from build123d import *

# Parameters (mm, degrees)
SZKIC1_R                    = 2.1
DODANIE_WYCI_GNI_CIE1_DEPTH = 24
WYTNIJ_WYCI_GNI_CIE1_REACH  = 31.306
SZKIC3_R                    = 3.45
WYTNIJ_WYCI_GNI_CIE2_DEPTH  = 4


with BuildPart() as part:
    # Szkic1 → Dodanie-wyciągnięcie1 (new body)
    with BuildSketch(Plane(origin=(0, 0, 0), x_dir=(1, 0, 0), z_dir=(0, 1, 0))):
        Polygon((12.5, 3.9), (-12.5, 3.9), (-14.9, 1.5), (-14.9, -1.5), (-12.5, -3.9), (12.5, -3.9), (14.9, -1.5), (14.9, 1.5), align=None)
        with Locations(Location((-11, 0, 0), (0, 0, 270))):
            Circle(SZKIC1_R, mode=Mode.SUBTRACT)
        with Locations(Location((11, 0, 0), (0, 0, 90))):
            Circle(SZKIC1_R, mode=Mode.SUBTRACT)
    extrude(amount=-DODANIE_WYCI_GNI_CIE1_DEPTH)

    # Szkic2 → Wytnij-wyciągnięcie1 (cut, up to next)
    with BuildSketch(Plane(origin=(0, 0, -3.9), x_dir=(-1, 0, 0), z_dir=(0, 0, -1)), mode=Mode.PRIVATE) as wytnij_wyci_gni_cie1_sk1:
        with BuildLine():
            Line((-7.1, -24), (7.1, -24))
            ThreePointArc((7.1, -24), (0, -16.9), (-7.1, -24))
        make_face()
    wytnij_wyci_gni_cie1_tool1 = extrude(wytnij_wyci_gni_cie1_sk1.sketch, amount=-WYTNIJ_WYCI_GNI_CIE1_REACH, mode=Mode.PRIVATE) & part.part
    add(wytnij_wyci_gni_cie1_tool1.solids().sort_by_distance((0, -20.986666, -3.9))[0], mode=Mode.SUBTRACT)

    # Szkic3 → Wytnij-wyciągnięcie2 (cut)
    with BuildSketch(Plane(origin=(0, 0, 0), x_dir=(1, 0, 0), z_dir=(0, 1, 0))):
        with Locations(Location((-11, 0, 0), (0, 0, 270))):
            Circle(SZKIC3_R)
        with Locations(Location((11, 0, 0), (0, 0, 90))):
            Circle(SZKIC3_R)
    extrude(amount=-WYTNIJ_WYCI_GNI_CIE2_DEPTH, mode=Mode.SUBTRACT)


solid = part.part
CAD build for the part. Positions are in the model's coordinates, mm. A direction names the side the tool comes from. Give positions to 0.01 mm unless a question says otherwise; leave off trailing zeros. Loops run counter-clockwise (first coordinate to the right, second up) from the corner with the lowest first, then second, coordinate; pieces in that order, holes last. Notation, with made-up numbers: M -8,35.5 L 25,35.5 A31 ccw 25,66.5 Z; hole C 69,40.5 d4. An arc over 180 degrees is marked long. One line per question, with ' | ' between items. Start each with the question number.
1. Probe L1, parallel to X at y = -2.85, z = 0; L2, parallel to X at y = -11.5, z = 0; L3, parallel to X at y = -19, z = 0. List the from-to ranges inside material, lowest first. Write a range as from..to.
2. Saw through at A-A on z = 0. Give the cut face in (x, y).
3. Saw through at B-B on x = 11. Give the cut face in (y, z), plus the area to 3 significant figures.
4. Saw through at D-D on x = -5. Give the cut face in (y, z), plus the area to 3 significant figures.
5. Two-plate mould, pull along Z, no slides. Class faces 1 (the face through (8.918, -13.86, 0.273)), 2 (the face through (13.7, -11.8, 2.7)), 3 (the face through (13.7, -11.8, -2.7)): pulls with the +Z half, pulls with the -Z half, needs draft (parallel to the pull), parting line crosses it, or undercut.
6. Flat gauge pins, fed straight in: pin 1 (1 mm diameter, centred on y = -17, z = -3, fed in from +X); pin 2 (2 mm diameter, centred on x = -11, z = 1.5, fed in from +Y); pin 3 (2.5 mm diameter, centred on x = 11, z = 0, fed in from +Y). Where does each tip first touch, or does it go through?
7. Saw through at C-C on y = -7. Give the cut face in (x, z), plus the area to 3 significant figures.
8. 3-axis set-ups, long thin cutter, end or side, ignore diameter. For faces 4 (the face through (-14.368, -1.972, -0.748)), 5 (the face through (-14.9, -12, 0)): which of +Z, -Z, +X, -X, +Y, -Y reach the whole face in a straight line?
Result sheet:
1) L1: x = -14.9..-14.45, -7.55..7.55, 14.45..14.9 | L2: x = -14.9..-13.1, -8.9..8.9, 13.1..14.9 | L3: x = -14.9..-13.1, -8.9..-5.04, 5.04..8.9, 13.1..14.9
2) outline: M -14.9,-24 L -13.1,-24 L -13.1,-4 L -14.45,-4 L -14.45,0 L -14.9,0 Z; M -8.9,-24 L -7.1,-24 A7.1 cw 7.1,-24 L 8.9,-24 L 8.9,-4 L 7.55,-4 L 7.55,0 L -7.55,0 L -7.55,-4 L -8.9,-4 Z; M 13.1,-24 L 14.9,-24 L 14.9,0 L 14.45,0 L 14.45,-4 L 13.1,-4 Z
3) outline: M -24,-3.9 L 0,-3.9 L 0,-3.45 L -4,-3.45 L -4,-2.1 L -24,-2.1 Z; M -24,2.1 L -4,2.1 L -4,3.45 L 0,3.45 L 0,3.9 L -24,3.9 Z | area: 75.6 mm^2
4) outline: M -18.96,-3.9 L 0,-3.9 L 0,3.9 L -18.96,3.9 Z | area: 148 mm^2
5) face 1: undercut | face 2: pulls with the +Z half | face 3: pulls with the -Z half
6) pin 1: stops at x = 13.9 | pin 2: stops at y = -4 | pin 3: passes through
7) outline: M -14.9,-1.5 L -12.5,-3.9 L 12.5,-3.9 L 14.9,-1.5 L 14.9,1.5 L 12.5,3.9 L -12.5,3.9 L -14.9,1.5 Z; hole C -11,0 d4.2; hole C 11,0 d4.2 | area: 193 mm^2
8) face 4: +Y | face 5: +Z, -Z, -X, +Y, -Y
